```python
from build123d import *

# Parameters (mm, degrees)
SKETCH1_R                 = 30
BOSS_EXTRUDE1_DEPTH       = 10
SKETCH2_W                 = 80
SKETCH2_H                 = 10
BOSS_EXTRUDE2_DEPTH       = 70
SKETCH3_R                 = 30
BOSS_EXTRUDE3_DEPTH       = 10
F_6_0MM_DOWEL_HOLE2_D     = 6
M4X0_7_TAPPED_HOLE2_D     = 3.3
M4X0_7_TAPPED_HOLE2_DEPTH = 6
M4X0_7_TAPPED_HOLE2_TIP   = 0.991420021
F_6_0MM_DOWEL_HOLE4_D     = 6
M4X0_7_TAPPED_HOLE4_D     = 3.3
M4X0_7_TAPPED_HOLE4_DEPTH = 6
M4X0_7_TAPPED_HOLE4_TIP   = 0.991420021
FILLET1_R                 = 30
FILLET2_R                 = 2


with BuildPart() as part:
    # Sketch1 → Boss-Extrude1 (new body)
    with BuildSketch(Plane.XY):
        Circle(SKETCH1_R)
    extrude(amount=BOSS_EXTRUDE1_DEPTH)

    # Sketch2 → Boss-Extrude2 (add)
    with BuildSketch(Plane.XY.offset(10)):
        with Locations((-40, -25)):
            Rectangle(SKETCH2_W, SKETCH2_H)
    extrude(amount=-BOSS_EXTRUDE2_DEPTH)

    # Sketch3 → Boss-Extrude3 (add)
    with BuildSketch(Plane.ZY.offset(80)):
        with Locations((-25, 0)):
            Circle(SKETCH3_R)
    extrude(amount=-BOSS_EXTRUDE3_DEPTH)

    # Ø6.0mm Dowel Hole2 (through all)
    with Locations(Plane(origin=(0, 0, 0), x_dir=(-1, 0, 0), z_dir=(0, 0, -1))):
        with Locations((0, 0)):
            Hole(F_6_0MM_DOWEL_HOLE2_D / 2)

    # M4x0.7 Tapped Hole2
    with Locations(Plane(origin=(0, 0, 0), x_dir=(-1, 0, 0), z_dir=(0, 0, -1))):
        with Locations((-15.5, 15.5), (15.5, 15.5), (15.5, -15.5), (-15.5, -15.5)):
            Hole(M4X0_7_TAPPED_HOLE2_D / 2, depth=M4X0_7_TAPPED_HOLE2_DEPTH)
            with Locations((0, 0, -(M4X0_7_TAPPED_HOLE2_DEPTH + M4X0_7_TAPPED_HOLE2_TIP / 2))):  # 118° drill point
                Cone(0, M4X0_7_TAPPED_HOLE2_D / 2, M4X0_7_TAPPED_HOLE2_TIP, mode=Mode.SUBTRACT)

    # Ø6.0mm Dowel Hole4 (through all)
    with Locations(Plane(origin=(-70, 1.407077757, -22.469041667), x_dir=(0, 0, -1), z_dir=(1, 0, 0))):
        with Locations((0, 0)):
            Hole(F_6_0MM_DOWEL_HOLE4_D / 2)

    # M4x0.7 Tapped Hole4
    with Locations(Plane(origin=(-70, 1.407077757, -22.469041667), x_dir=(0, 0, -1), z_dir=(1, 0, 0))):
        with Locations((-15.5, 15.5), (15.5, 15.5), (15.5, -15.5), (-15.5, -15.5)):
            Hole(M4X0_7_TAPPED_HOLE4_D / 2, depth=M4X0_7_TAPPED_HOLE4_DEPTH)
            with Locations((0, 0, -(M4X0_7_TAPPED_HOLE4_DEPTH + M4X0_7_TAPPED_HOLE4_TIP / 2))):  # 118° drill point
                Cone(0, M4X0_7_TAPPED_HOLE4_D / 2, M4X0_7_TAPPED_HOLE4_TIP, mode=Mode.SUBTRACT)

    # Fillet1
    fillet1_edges = [part.edges().sort_by_distance(p)[0] for p in [
        (0, -25, -60),
    ]]
    fillet(fillet1_edges, radius=FILLET1_R)

    # Fillet2
    fillet2_edges = [part.edges().sort_by_distance(p)[0] for p in [
        (-80, -20, -53.680339887),
        (-51.180339887, -20, 10),
        (-80, -20, 3.680339887),
        (0, -20, -15),
        (-55, -20, -60),
        (-8.786796564, -20, -51.213203436),
    ]]
    fillet(fillet2_edges, radius=FILLET2_R)


solid = part.part
```
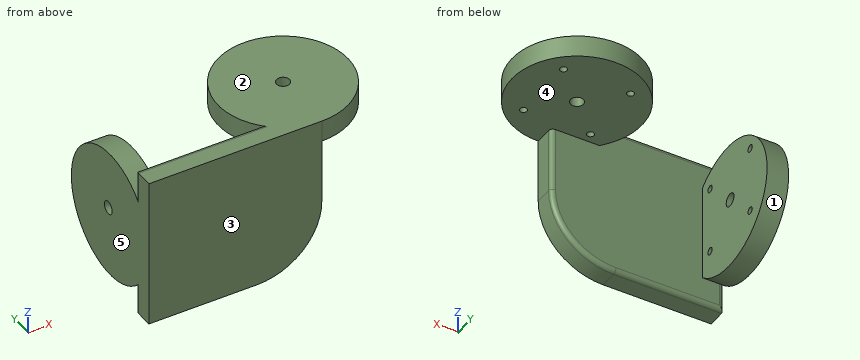
Here's how the part is built. I have some questions about the finished solid (model axes, mm). Face numbers are marked on the shaded views. A direction names the side the tool comes from. Coordinates: 2 decimals unless noted, no trailing zeros. Order: outer loops, then holes, each group sorted by start corner. A loop starts at its lowest first (then second) coordinate and runs counter-clockwise, first axis right, second up.
Item 1: If we section it at A-A, the plane x = -72.5: List the corners of the cut face in (y, z) for me, then the cut area to 3 significant figures.
Response values:
outline: (-30, -60) - (-22, -60) arc R2 ccw to (-20, -58) - (-20, -47.36) arc R30 ccw (long way) to (-20, -2.64) - (-20, 8) arc R2 ccw to (-22, 10) - (-30, 10) - close; hole circle Ø3.3 at (-14.09, -37.97); hole circle Ø3.3 at (-14.09, -6.97); hole circle Ø6 at (1.41, -22.47); hole circle Ø3.3 at (16.91, -37.97); hole circle Ø3.3 at (16.91, -6.97)
area: 3,150 mm2
Item 2: If we section it at B-B, the plane y = 0: List the corners of the cut face in (x, z) for me, then the cut area to 3 significant figures.
Response values:
outline: (-80, -55) - (-70, -55) - (-70, -25.12) - (-80, -25.12) - close; (-80, -19.82) - (-70, -19.82) - (-70, 5) - (-80, 5) - close; (-30, 0) - (-3, 0) - (-3, 10) - (-30, 10) - close; (3, 0) - (30, 0) - (30, 10) - (3, 10) - close
area: 1,090 mm2
Item 3: Thinking about a two-plate mould opening in Y: for the marked faces 1, 2 and 3, which applies, pulls with the +Y half, pulls with the -Y half, needs draft (parallel to the pull), parting line crosses it, or undercut?
Response values:
face 1: undercut
face 2: needs draft
face 3: pulls with the -Y half
Item 4: If we section it at C-C, the plane x = -46.5: List the corners of the cut face in (y, z) for me.
Response values:
outline: (-30, -60) - (-22, -60) arc R2 ccw to (-20, -58) - (-20, 8) arc R2 ccw to (-22, 10) - (-30, 10) - close
Item 5: I'm going to push flat-ended pins straight in: pin 1 Ø4.5 at (y, z) = (16.91, -37.97) entering from +X; pin 2 Ø3 at (y, z) = (-14.09, -37.97) entering from +X; pin 3 Ø3.5 at (x, y) = (0, 0) entering from +Z; pin 4 Ø6.5 at (y, z) = (-25.5, -16.5) entering from +X. Where does each tip first touch, or does it pass through?
Response values:
pin 1: stops at x = -70
pin 2: stops at x = -76.09
pin 3: passes through
pin 4: stops at x = 0
Item 6: I need wall thicknesses on probe 1 along Y at (x, z) = (0, 3.75); probe 2 along Y at (x, z) = (15, 1). Which ranges of each line are inside material? Lowest first, please.
Response values:
probe 1: y = -30 to -3, 3 to 30
probe 2: y = -25.98 to -17.07, -13.93 to 13.93, 17.07 to 25.98
Item 7: Which directions (+Z, -Z, +X, -X, +Y, -Y) give clear straight access to the entire face, cutting with the end or side of a thin tool? Please do the marked faces 4 and 5.
Response values:
face 4: -Z, +X, +Y
face 5: +Z, -Z, -X, +Y, -Y
